```python
from build123d import *

# Parameters (mm, degrees)
SKETCH1_W           = 70
SKETCH1_H           = 36
BOSS_EXTRUDE1_DEPTH = 1
FILLET1_R           = 1


with BuildPart() as part:
    # Sketch1 → Boss-Extrude1 (new body)
    with BuildSketch(Plane(origin=(0, 0, 0), x_dir=(1, 0, 0), z_dir=(0, 1, 0))):
        with BuildLine():
            Line((-35, 25), (-35, 18))
            Line((-35, 18), (-35, -18))
            Line((-35, -18), (-35, -25))
            ThreePointArc((-35, -25), (-60, 0), (-35, 25))
        make_face()
        Rectangle(SKETCH1_W, SKETCH1_H)
    extrude(amount=BOSS_EXTRUDE1_DEPTH)

    # Fillet1
    fillet1_edges = [part.edges().sort_by_distance(p)[0] for p in [
        (-35, 0.5, -18),
        (-35, 0.5, 18),
        (-35, 0.5, 25),
        (-35, 0.5, -25),
    ]]
    fillet(fillet1_edges, radius=FILLET1_R)


solid = part.part
```
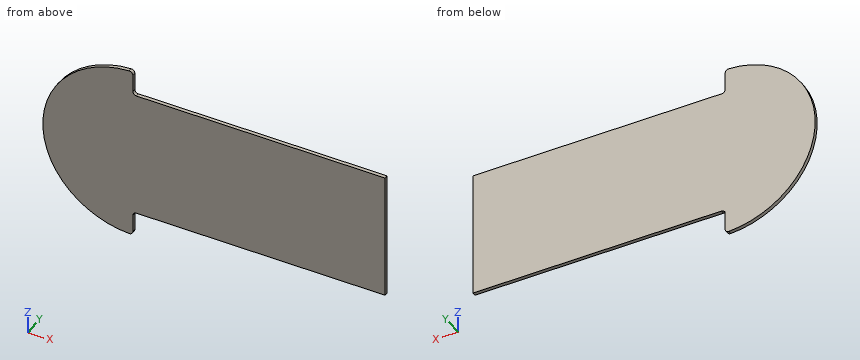
Can you work these out from the model? Positions are in its coordinate system, mm. Coordinates: 2 decimals unless noted, no trailing zeros. Loops run counter-clockwise (first coordinate to the right, second up) from the corner with the lowest first, then second, coordinate; pieces in that order, holes last. Notation, with made-up numbers: (78.5, -27.5) -> (92.5, -27.5) arc R32 ccw to (92.5, 8.5) -> close; hole circle Ø6 at (-32, -1.75). An arc over 180 degrees is marked (long way). Answer as a JSON object with one key per item and string values.
1) Imagine slicing it at A-A (y = 0.25). Please give me the cut outline in (x, z).
Results:
{"outline": "(-36.04, -24.98) arc R1 ccw to (-35, -23.98) -> (-35, -19) arc R1 cw to (-34, -18) -> (35, -18) -> (35, 18) -> (-34, 18) arc R1 cw to (-35, 19) -> (-35, 23.98) arc R1 ccw to (-36.04, 24.98) arc R25 ccw to start"}
2) If I drill on line 1 (Z direction, x = -14, y = 0.5); line 2 (X direction, y = 0.3, z = -0.5) (3 decimals); line 3 (Z direction, x = -36.5, y = 0.2), over which ranges is the centre line in solid material (lowest first)?
Results:
{"line 1": "z = -18 to 18", "line 2": "x = -59.995 to 35", "line 3": "z = -24.95 to 24.95"}
3) Imagine slicing it at B-B (z = -15). Please give me the cut outline in (x, y).
Results:
{"outline": "(-55, 0) -> (35, 0) -> (35, 1) -> (-55, 1) -> close"}
4) Imagine slicing it at C-C (x = -3.5). Please give me the cut outline in (y, z).
Results:
{"outline": "(0, -18) -> (1, -18) -> (1, 18) -> (0, 18) -> close"}
